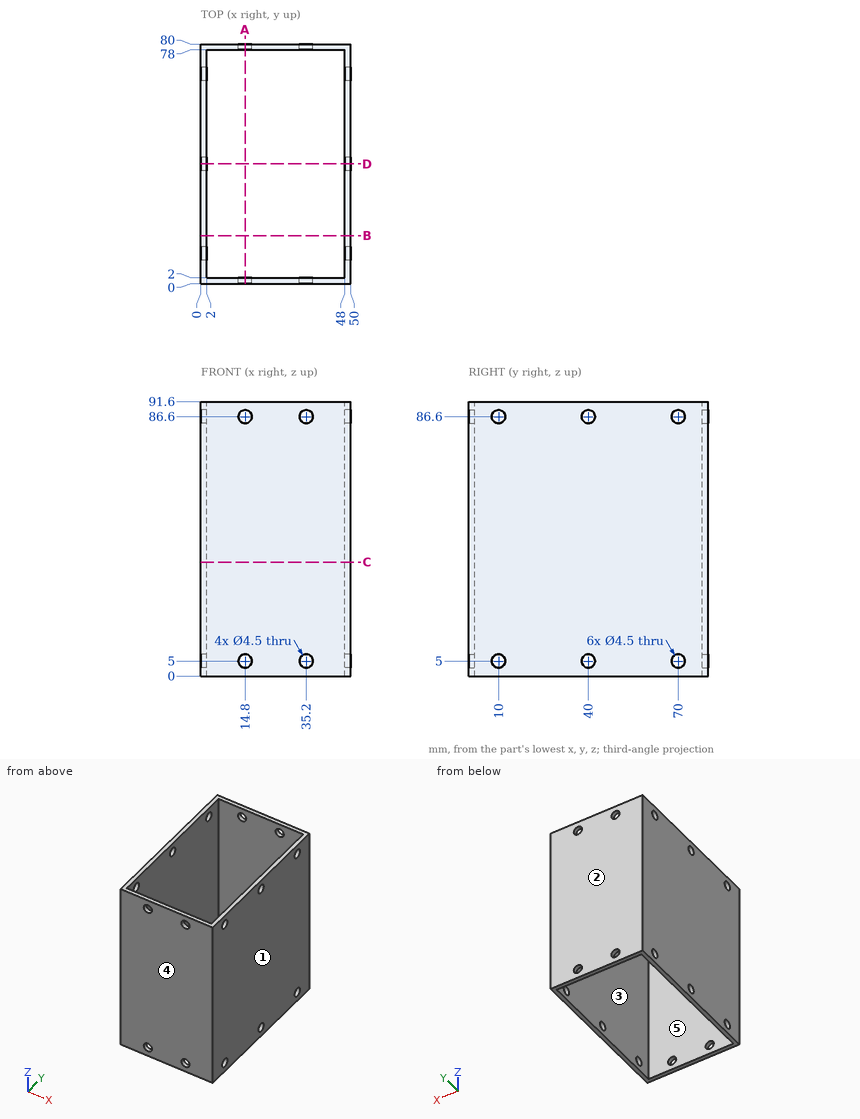
Check sheet for the drawn part. Datum: minimum x, y, z corner. Units: mm. A direction names the side the tool comes from. Round coordinates to 2 decimals unless told otherwise and drop trailing zeros. Loops run counter-clockwise (first coordinate to the right, second up) from the corner with the lowest first, then second, coordinate; pieces in that order, holes last. Notation, with made-up numbers: M 27.5,-24 L 65.5,-24 A13 cw 65.5,-8 Z; hole C 67,61.25 d4. An arc over 180 degrees is marked long. Write each question's results on one line, items separated by ' | '.
1) Gauge pin test, flat end, axial feed: P1, Ø12, axis at x = 36.5, y = 38.5, coming from the +Z side. Record the tip position at first contact, or that the pin passes through.
Checks:
P1: passes through
2) Access from +Z, -Z, +X, -X, +Y, -Y to the whole of each face (thin tool, end or side, straight path). Record for the marked faces 4 and 5.
Checks:
face 4: +Z, -Z, +X, -X, -Y | face 5: +Z, -Z
3) Scan lines: L1, parallel to Z at x = 49, y = 70; L2, parallel to Y at x = 1.1, z = 5; L3, parallel to X at y = 0.5, z = 86.6. Record each from-to range of solid material in increasing order. Write a range as from..to.
Checks:
L1: z = 0..2.75, 7.25..84.35, 88.85..91.6 | L2: y = 0..7.75, 12.25..37.75, 42.25..67.75, 72.25..80 | L3: x = 0..12.55, 17.05..32.95, 37.45..50
4) Section check C-C on z = 38. Record the boundary of the cut face in (x, y).
Checks:
outline: M 0,0 L 50,0 L 50,80 L 0,80 Z; hole M 2,2 L 48,2 L 48,78 L 2,78 Z
5) Section check B-B on y = 16. Record the boundary of the cut face in (x, z).
Checks:
outline: M 0,0 L 2,0 L 2,91.6 L 0,91.6 Z; M 48,0 L 50,0 L 50,91.6 L 48,91.6 Z
6) Section check D-D on y = 40. Record the boundary of the cut face in (x, z), then the cut area to 3 significant figures.
Checks:
outline: M 0,0 L 2,0 L 2,2.75 L 0,2.75 Z; M 0,7.25 L 2,7.25 L 2,84.35 L 0,84.35 Z; M 0,88.85 L 2,88.85 L 2,91.6 L 0,91.6 Z; M 48,0 L 50,0 L 50,2.75 L 48,2.75 Z; M 48,7.25 L 50,7.25 L 50,84.35 L 48,84.35 Z; M 48,88.85 L 50,88.85 L 50,91.6 L 48,91.6 Z | area: 330 mm2
7) Section check A-A on x = 14.8. Record the boundary of the cut face in (y, z).
Checks:
outline: M 0,0 L 2,0 L 2,2.75 L 0,2.75 Z; M 0,7.25 L 2,7.25 L 2,84.35 L 0,84.35 Z; M 0,88.85 L 2,88.85 L 2,91.6 L 0,91.6 Z; M 78,0 L 80,0 L 80,2.75 L 78,2.75 Z; M 78,7.25 L 80,7.25 L 80,84.35 L 78,84.35 Z; M 78,88.85 L 80,88.85 L 80,91.6 L 78,91.6 Z
8) Mould release check, pull along Y, two halves, no side actions. Record for the marked faces 1, 2 and 3: released by +Y, released by -Y, zero draft, split by the parting line, or undercut.
Checks:
face 1: zero draft | face 2: released by +Y | face 3: undercut
